Answer from the drawing. Dimensions are ordinates in mm from the lowest x, y and z of the part. Give positions to 0.01 mm unless a question says otherwise; leave off trailing zeros. Order: outer loops, then holes, each group sorted by start corner. A loop starts at its lowest first (then second) coordinate and runs counter-clockwise, first axis right, second up. Notation, with made-up numbers: (1, 9.25) - (18, 9.25) arc R19 cw to (18, 45.25) - close; hole circle Ø2 at (66, 74). An arc over 180 degrees is marked (long way). Answer in a Markdown table with one row per item. Add a question column.
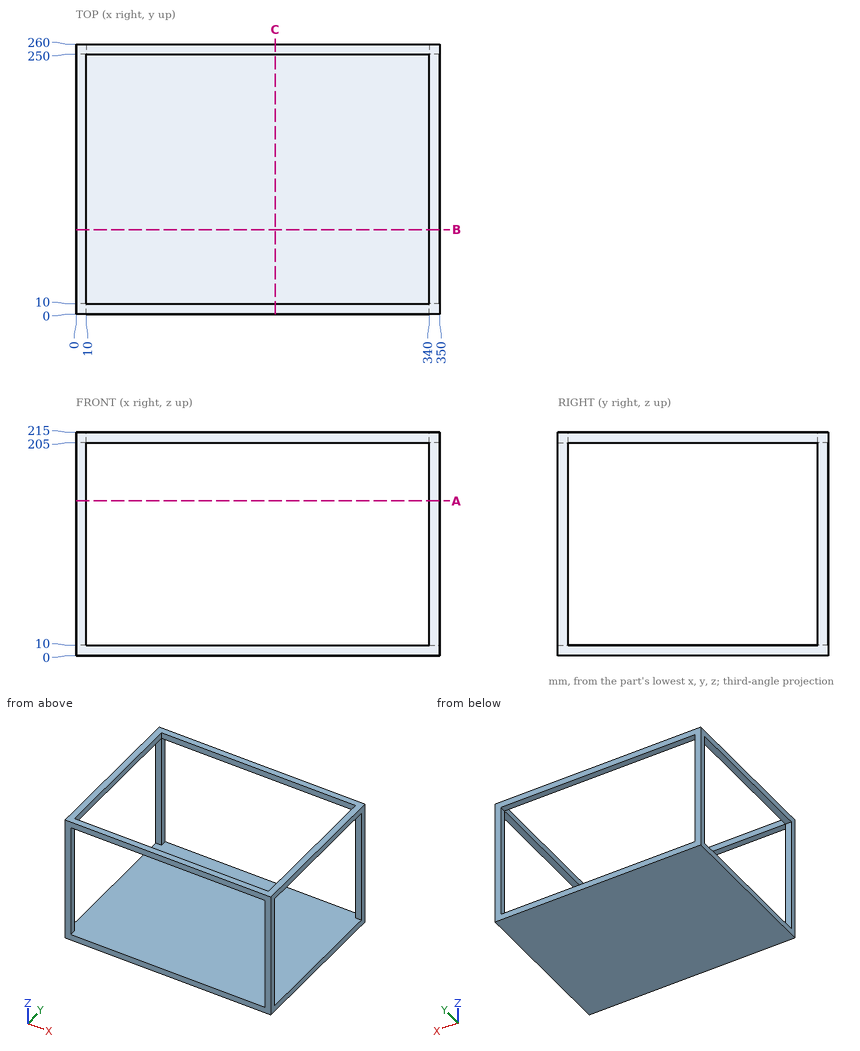
(1) A straight line is drawn through the part: line 1 (Z direction, x = 50, y = 106.5). Find the intervals that lie inside material, in ascending order.
(2) Find section C-C, the plane x = 191.5. Write down the section's boundary in (y, z).
(3) This flat-tipped pin is pushed along its axis until it touches: P1, Ø1.5, axis at x = 230.5, y = 147, coming from the +Z side. Where does it stop, or does it pass through?
(4) Find section B-B, the plane y = 81.5. Write down the section's boundary in (x, z), plus the area to 3 significant figures.
(5) Find section A-A, the plane z = 149. Write down the section's boundary in (x, y).
Answer key:
| question | item | result |
|---|---|---|
| 1 | line 1 | 0 to 10 |
| 2 | outline | (0, 0) - (260, 0) - (260, 10) - (0, 10) - close; (0, 205) - (10, 205) - (10, 215) - (0, 215) - close; (250, 205) - (260, 205) - (260, 215) - (250, 215) - close |
| 3 | P1 | z = 10 |
| 4 | outline | (0, 0) - (350, 0) - (350, 10) - (0, 10) - close; (0, 205) - (10, 205) - (10, 215) - (0, 215) - close; (340, 205) - (350, 205) - (350, 215) - (340, 215) - close |
| 4 | area | 3,700 mm² |
| 5 | outline | (0, 0) - (10, 0) - (10, 10) - (0, 10) - close; (0, 250) - (10, 250) - (10, 260) - (0, 260) - close; (340, 0) - (350, 0) - (350, 10) - (340, 10) - close; (340, 250) - (350, 250) - (350, 260) - (340, 260) - close |
